from build123d import *

# Parameters (mm, degrees)
SKETCH1_W               = 2362.2
SKETCH1_H               = 609.6
SKETCH1_R               = 13.119830451
SKETCH1_W_2             = 50.8
SKETCH1_H_2             = 50.8
BOSS_EXTRUDE1_DEPTH     = 101.6
SKETCH2_W               = 127
SKETCH2_H               = 63.5
CUT_EXTRUDE1_DEPTH      = 50.8
SKETCH3_R               = 4.7625
CUT_EXTRUDE2_DEPTH      = 152.4
SKETCH4_W               = 76.2
SKETCH4_H               = 34.925
CUT_EXTRUDE3_DEPTH      = 1334.016102678
CUT_EXTRUDE4_DEPTH      = 2384.94933671
CUT_EXTRUDE4_DEPTH_BACK = 352.425
SKETCH5_W               = 6.35
SKETCH5_H               = 19.05
SKETCH6_W               = 101.6
SKETCH6_H               = 103.1875
CUT_EXTRUDE5_DEPTH      = 76.2
SKETCH7_R               = 4.7625
CUT_EXTRUDE6_DEPTH      = 1222.6160631
SKETCH9_W               = 1704.975
SKETCH9_H               = 44.45
CUT_EXTRUDE7_DEPTH      = 1225.019121583


with BuildPart() as part:
    # Sketch1 → Boss-Extrude1 (new body)
    with BuildSketch(Plane.XY):
        Rectangle(SKETCH1_W, SKETCH1_H)
        with Locations((-952.5, 139.7)):
            Circle(SKETCH1_R, mode=Mode.SUBTRACT)
        with Locations((-647.7, 215.9)):
            Circle(SKETCH1_R, mode=Mode.SUBTRACT)
        with Locations((-266.7, 215.9)):
            Circle(SKETCH1_R, mode=Mode.SUBTRACT)
        with Locations((114.3, 215.9)):
            Circle(SKETCH1_R, mode=Mode.SUBTRACT)
        with Locations((495.3, 215.9)):
            Circle(SKETCH1_R, mode=Mode.SUBTRACT)
        with Locations((-901.7, -114.3)):
            Rectangle(SKETCH1_W_2, SKETCH1_H_2, mode=Mode.SUBTRACT)
    extrude(amount=BOSS_EXTRUDE1_DEPTH)

    # Sketch2 → Cut-Extrude1 (cut)
    with BuildSketch(Plane(origin=(0, 0, 0), x_dir=(-1, 0, 0), z_dir=(0, 0, -1))):
        with Locations((736.6, 241.3)):
            Rectangle(SKETCH2_W, SKETCH2_H)
        with Locations((736.6, -241.3)):
            Rectangle(SKETCH2_W, SKETCH2_H)
        with Locations((-812.8, 241.3)):
            Rectangle(SKETCH2_W, SKETCH2_H)
        with Locations((-812.8, -241.3)):
            Rectangle(SKETCH2_W, SKETCH2_H)
    extrude(amount=-CUT_EXTRUDE1_DEPTH, mode=Mode.SUBTRACT)

    # Sketch3 → Cut-Extrude2 (cut)
    with BuildSketch(Plane.XZ.offset(304.8)):
        with Locations((844.55, 25.4)):
            Circle(SKETCH3_R)
        with Locations((781.05, 25.4)):
            Circle(SKETCH3_R)
        with Locations((-704.85, 25.4)):
            Circle(SKETCH3_R)
        with Locations((-768.35, 25.4)):
            Circle(SKETCH3_R)
    extrude(amount=-CUT_EXTRUDE2_DEPTH, mode=Mode.SUBTRACT)

    # Sketch4 → Cut-Extrude3 (cut, through all)
    with BuildSketch(Plane.XZ.offset(304.8)):
        with Locations((1143, 17.4625)):
            Rectangle(SKETCH4_W, SKETCH4_H)
        with Locations((1143, 84.1375)):
            Rectangle(SKETCH4_W, SKETCH4_H)
    extrude(amount=-CUT_EXTRUDE3_DEPTH, mode=Mode.SUBTRACT)

    # Sketch5 → Cut-Extrude4 (cut, two sides: drawn at the far end of the back side and taken through both)
    # profile 1 of 4: a face of its own
    with BuildSketch(Plane(origin=(1181.1, 0, 0), x_dir=(0, 0, -1), z_dir=(1, 0, 0)).offset(-CUT_EXTRUDE4_DEPTH_BACK)):
        with Locations((-3.175, -149.225)):
            Rectangle(SKETCH5_W, SKETCH5_H)
    # profile 2 of 4: a face of its own
    with BuildSketch(Plane(origin=(1181.1, 0, 0), x_dir=(0, 0, -1), z_dir=(1, 0, 0)).offset(-CUT_EXTRUDE4_DEPTH_BACK)):
        Polygon((-6.35, -139.7), (0, -139.7), (0, -36.5125), (-6.35, -36.5125), (-53.975, -36.5125), (-53.975, -77.7875), (-53.975, -95.25), (-101.6, -95.25), (-101.6, -139.7), align=None)
        with BuildLine():
            ThreePointArc((-12.7, -77.7875), (-31.75, -96.8375), (-50.8, -77.7875))
            ThreePointArc((-50.8, -77.7875), (-31.75, -58.7375), (-12.7, -77.7875))
        make_face(mode=Mode.SUBTRACT)
    # profile 3 of 4: a face of its own
    with BuildSketch(Plane(origin=(1181.1, 0, 0), x_dir=(0, 0, -1), z_dir=(1, 0, 0)).offset(-CUT_EXTRUDE4_DEPTH_BACK)):
        with BuildLine():
            ThreePointArc((-12.7, -77.7875), (-31.75, -58.7375), (-50.8, -77.7875))
            ThreePointArc((-50.8, -77.7875), (-31.75, -96.8375), (-12.7, -77.7875))
        make_face()
    # profile 4 of 4: a face of its own
    with BuildSketch(Plane(origin=(1181.1, 0, 0), x_dir=(0, 0, -1), z_dir=(1, 0, 0)).offset(-CUT_EXTRUDE4_DEPTH_BACK)):
        with Locations((-3.175, -26.9875)):
            Rectangle(SKETCH5_W, SKETCH5_H)
    extrude(amount=CUT_EXTRUDE4_DEPTH + CUT_EXTRUDE4_DEPTH_BACK, mode=Mode.SUBTRACT)

    # Sketch6 → Cut-Extrude5 (cut)
    with BuildSketch(Plane(origin=(1181.1, 0, 0), x_dir=(0, 0, -1), z_dir=(1, 0, 0))):
        with Locations((-50.8, -88.10625)):
            Rectangle(SKETCH6_W, SKETCH6_H)
    extrude(amount=-CUT_EXTRUDE5_DEPTH, mode=Mode.SUBTRACT)

    # Sketch7 → Cut-Extrude6 (cut, through all)
    with BuildSketch(Plane.XY.offset(66.675)):
        with Locations((1143, 266.7)):
            Circle(SKETCH7_R)
        with Locations((1143, 133.35)):
            Circle(SKETCH7_R)
        with Locations((1143, 0)):
            Circle(SKETCH7_R)
        with Locations((1143, -266.7)):
            Circle(SKETCH7_R)
    extrude(amount=-CUT_EXTRUDE6_DEPTH, mode=Mode.SUBTRACT)

    # Sketch9 → Cut-Extrude7 (cut, through all)
    with BuildSketch(Plane.XY.offset(101.6)):
        with Locations((-23.8125, -117.475)):
            Rectangle(SKETCH9_W, SKETCH9_H)
    extrude(amount=-CUT_EXTRUDE7_DEPTH, mode=Mode.SUBTRACT)


solid = part.part
Build history of the part. All positions in model axes, mm. A direction names the side the tool comes from. Give positions to 0.01 mm unless a question says otherwise; leave off trailing zeros. Loops run counter-clockwise (first coordinate to the right, second up) from the corner with the lowest first, then second, coordinate; pieces in that order, holes last. Notation, with made-up numbers: (0, 22) -> (11, 22) arc R27 ccw to (11, 44) -> close; hole circle Ø10 at (31.5, -28). An arc over 180 degrees is marked (long way). Answer in a Markdown table with one row per item.
Item 1: Flat gauge pins, fed straight in: P1, Ø15, axis at y = -121.5, z = 37.5, coming from the +X side; P2, Ø15, axis at y = -244, z = 22, coming from the +X side; P3, Ø11, axis at x = 1143, y = 0, coming from the -Z side (3 decimals). Where does each tip first touch, or does it go through?
Findings below:
| item | result |
|---|---|
| P1 | stops at x = -927.1 |
| P2 | stops at x = 1104.9 |
| P3 | stops at z = 34.925 |
Item 2: Slice it at C-C on x = 345.5. Write the cut outline in (y, z), plus the area to 3 significant figures.
Findings below:
| item | result |
|---|---|
| outline | (-304.8, 0) -> (-139.7, 0) -> (-139.7, 101.6) -> (-304.8, 101.6) -> close; (-95.25, 0) -> (304.8, 0) -> (304.8, 101.6) -> (-95.25, 101.6) -> close |
| area | 57,400 mm² |
Item 3: Mould opens along X. For faces 1 (the flat face through (965, -65, 53.975)), 2 (the flat face through (-800.1, -242, 25)), 3 (the flat face through (814, 273.05, 25)) say: pulls with the +X half, pulls with the -X half, needs draft (parallel to the pull), parting line crosses it, or undercut.
Findings below:
| item | result |
|---|---|
| face 1 | needs draft |
| face 2 | undercut |
| face 3 | undercut |
Item 4: Slice it at B-B on y = 98.5. Write the cut outline in (x, z) (3 decimals).
Findings below:
| item | result |
|---|---|
| outline | (-1181.1, 0) -> (1104.9, 0) -> (1104.9, 34.925) -> (1181.1, 34.925) -> (1181.1, 66.675) -> (1104.9, 66.675) -> (1104.9, 101.6) -> (-1181.1, 101.6) -> close |
Item 5: Slice it at D-D on y = -118. Write the cut outline in (x, z).
Findings below:
| item | result |
|---|---|
| outline | (-1181.1, 0) -> (-927.1, 0) -> (-927.1, 101.6) -> (-1181.1, 101.6) -> close |
Item 6: Tool access for faces 4 (the flat face through (-673.1, 241, 25)), 5 (the flat face through (-902, -88.9, 50)), 6 (the flat face through (1134, 132, 34.925)): list every direction of +Z, -Z, +X, -X, +Y, -Y with a clear straight run to the whole face (end or side of a thin tool).
Findings below:
| item | result |
|---|---|
| face 4 | -Z |
| face 5 | +Z, -Z |
| face 6 | -Z, +X, +Y, -Y |
Item 7: Probe line 1 along Y through (x, z) = (-647.7, 28.5); line 2 along X through (y, z) = (-266.7, 46.5); line 3 along X through (y, z) = (-266, 42). List the from-to ranges inside material, lowest first. Write a range as [from, to].
Findings below:
| item | result |
|---|---|
| line 1 | y = [-304.8, -139.7], [-95.25, 202.78], [229.02, 304.8] |
| line 2 | x = [-1181.1, -800.1], [-673.1, 749.3], [876.3, 1138.24], [1147.76, 1181.1] |
| line 3 | x = [-1181.1, -800.1], [-673.1, 749.3], [876.3, 1138.29], [1147.71, 1181.1] |
